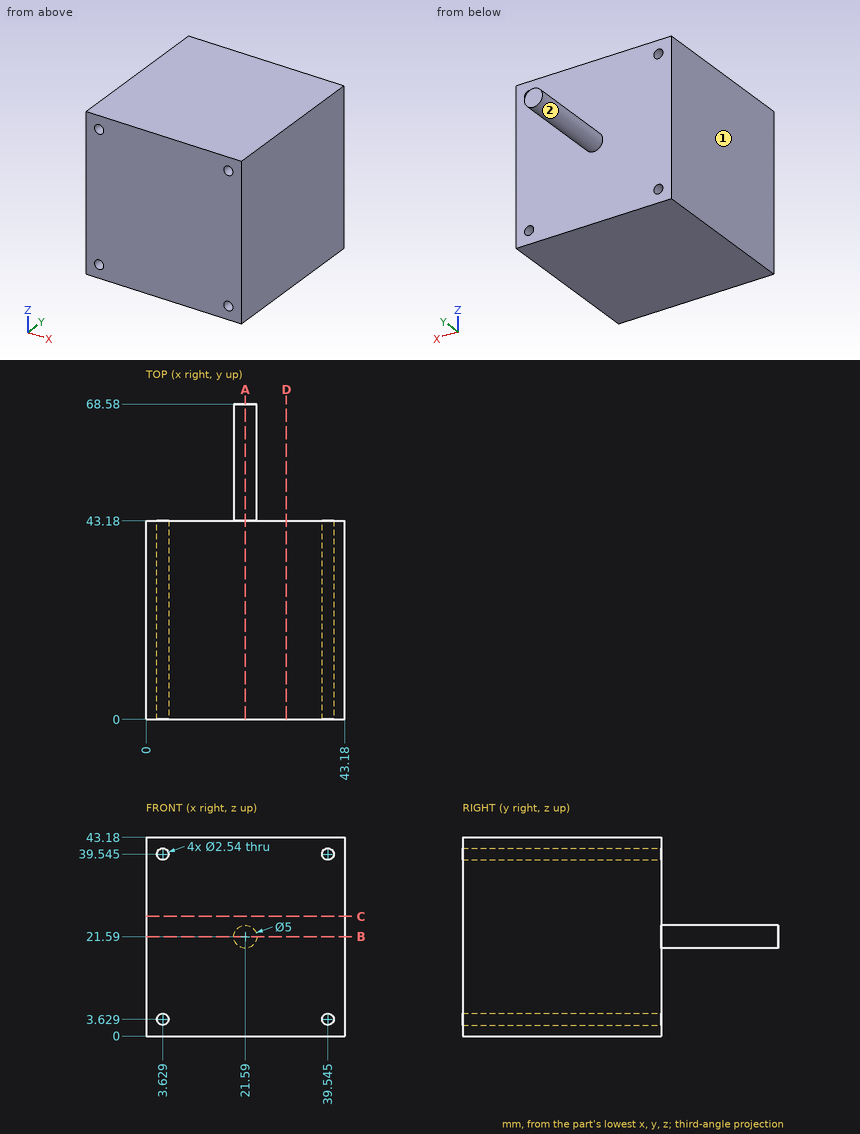
The drawing under review shows one solid part. Ordinate dimensions are in mm from its lowest x, y, z. A direction names the side the tool comes from. Round coordinates to 2 decimals unless told otherwise and drop trailing zeros. Loops run counter-clockwise (first coordinate to the right, second up) from the corner with the lowest first, then second, coordinate; pieces in that order, holes last. Notation, with made-up numbers: (-4.5, 37) - (33.5, 37) arc R26 ccw to (33.5, 54) - close; hole circle Ø2 at (6, -30.75). An arc over 180 degrees is marked (long way). Use a Markdown table: item, result. Add a question column.
Q1. Add section B-B (z = 21.59). State the section outline as (x, y) points, plus the area to 3 significant figures.
Q2. For probe 1 along X at (y, z) = (16, 3.5) (1 decimal); probe 2 along Y at (x, z) = (35, 31); probe 3 along Z at (x, y) = (4.5, 14.5) (1 decimal), list the stretches that pass through material, from the lowest coordinate up.
Q3. Machinability: for the marked faces 1 and 2, which of the approach directions +Z, -Z, +X, -X, +Y, -Y give a long, thin tool a straight path to every point of the face, cutting with its end or side? Answer none if there is none.
Q4. Insertion check: pin 1 Ø4 at (x, z) = (3.63, 39.55) entering from +Y; pin 2 Ø2 at (x, z) = (39.55, 39.55) entering from -Y; pin 3 Ø6 at (y, z) = (9, 9.5) entering from -X. Each pin has a flat end and moves straight along its axis. Give the tip position at first contact, or say it passes through.
Q5. Add section C-C (z = 26). State the section outline as (x, y) points, plus the area to 3 significant figures.
Q6. Add section A-A (x = 21.59). State the section outline as (y, z) points.
Worked answers:
| question | item | result |
|---|---|---|
| 1 | outline | (0, 0) - (43.18, 0) - (43.18, 43.18) - (24.09, 43.18) - (24.09, 68.58) - (19.09, 68.58) - (19.09, 43.18) - (0, 43.18) - close |
| 1 | area | 1,990 mm² |
| 2 | probe 1 | 0 to 2.4, 4.9 to 38.3, 40.8 to 43.2 |
| 2 | probe 2 | 0 to 43.18 |
| 2 | probe 3 | 0 to 2.7, 4.6 to 38.6, 40.5 to 43.2 |
| 3 | face 1 | +Z, -Z, -X, +Y, -Y |
| 3 | face 2 | +Y |
| 4 | pin 1 | y = 43.18 |
| 4 | pin 2 | through |
| 4 | pin 3 | x = 0 |
| 5 | outline | (0, 0) - (43.18, 0) - (43.18, 43.18) - (0, 43.18) - close |
| 5 | area | 1,860 mm² |
| 6 | outline | (0, 0) - (43.18, 0) - (43.18, 19.09) - (68.58, 19.09) - (68.58, 24.09) - (43.18, 24.09) - (43.18, 43.18) - (0, 43.18) - close |
